Build history of the part. All positions in model axes, mm. A direction names the side the tool comes from. Round coordinates to 2 decimals unless told otherwise and drop trailing zeros. Write each loop counter-clockwise with the first axis right and the second up, starting at its lowest first coordinate (ties: lowest second). Pieces come first, ordered by that corner, then holes. Notation, with made-up numbers: (69, -11) - (75, -11) arc R26 ccw to (75, 5) - close; hole circle Ø11 at (-20, 34). An arc over 180 degrees is marked (long way). One line per question, with ' | ' between items.
from build123d import *

# Parameters (mm, degrees)
SKETCH1_W           = 1219.2
SKETCH1_H           = 508
BOSS_EXTRUDE1_DEPTH = 25.4
SKETCH2_W           = 50.8
SKETCH2_H           = 508
BOSS_EXTRUDE2_DEPTH = 304.8
SKETCH3_W           = 101.6
SKETCH3_H           = 50.8
BOSS_EXTRUDE3_DEPTH = 152.4


with BuildPart() as part:
    # Sketch1 → Boss-Extrude1 (new body)
    with BuildSketch(Plane(origin=(0, 0, 0), x_dir=(1, 0, 0), z_dir=(0, 1, 0))):
        with Locations((609.6, 254)):
            Rectangle(SKETCH1_W, SKETCH1_H)
    extrude(amount=BOSS_EXTRUDE1_DEPTH)

    # Sketch2 → Boss-Extrude2 (add)
    with BuildSketch(Plane(origin=(0, 25.4, 0), x_dir=(1, 0, 0), z_dir=(0, 1, 0))):
        with Locations((1193.8, 254)):
            Rectangle(SKETCH2_W, SKETCH2_H)
    extrude(amount=BOSS_EXTRUDE2_DEPTH)

    # Sketch3 → Boss-Extrude3 (add)
    with BuildSketch(Plane.XZ):
        with Locations((50.8, -25.4)):
            Rectangle(SKETCH3_W, SKETCH3_H)
        with Locations((50.8, -482.6)):
            Rectangle(SKETCH3_W, SKETCH3_H)
        with Locations((1168.4, -25.4)):
            Rectangle(SKETCH3_W, SKETCH3_H)
        with Locations((1168.4, -482.6)):
            Rectangle(SKETCH3_W, SKETCH3_H)
    extrude(amount=BOSS_EXTRUDE3_DEPTH)


solid = part.part
Q1. Saw through at A-A, the plane y = -114.5. List the corners of the cut face in (x, z), then the cut area to 3 significant figures.
Found:
outline: (0, -508) - (101.6, -508) - (101.6, -457.2) - (0, -457.2) - close; (0, -50.8) - (101.6, -50.8) - (101.6, 0) - (0, 0) - close; (1117.6, -508) - (1219.2, -508) - (1219.2, -457.2) - (1117.6, -457.2) - close; (1117.6, -50.8) - (1219.2, -50.8) - (1219.2, 0) - (1117.6, 0) - close | area: 20,600 mm^2
Q2. Saw through at C-C, the plane x = 364. List the corners of the cut face in (y, z), then the cut area to 3 significant figures.
Found:
outline: (0, -508) - (25.4, -508) - (25.4, 0) - (0, 0) - close | area: 12,900 mm^2
Q3. Which spindle directions (+Z, -Z, +X, -X, +Y, -Y) get a long thin tool onto all of the face, cutting with end or side? Do faces 4 (the flat face through (50, -75, -50.8)), 5 (the flat face through (1168.4, 176, -250)), 6 (the flat face through (101.6, -75, -483)). Say none if no direction does.
Found:
face 4: +X, -X, -Y | face 5: +Z, -Z, -X, +Y | face 6: +Z, -Z, -Y
Q4. Saw through at D-D, the plane y = 279. List the corners of the cut face in (x, z), then the cut area to 3 significant figures.
Found:
outline: (1168.4, -508) - (1219.2, -508) - (1219.2, 0) - (1168.4, 0) - close | area: 25,800 mm^2
Q5. Saw through at B-B, the plane z = -32. List the corners of the cut face in (x, y), then the cut area to 3 significant figures.
Found:
outline: (0, -152.4) - (101.6, -152.4) - (101.6, 0) - (1117.6, 0) - (1117.6, -152.4) - (1219.2, -152.4) - (1219.2, 330.2) - (1168.4, 330.2) - (1168.4, 25.4) - (0, 25.4) - close | area: 77,400 mm^2
Q6. Drop flat-ended pins along their axis: pin 1 (12 mm diameter, centred on x = 592, z = -457, fed in from +Y); pin 2 (5 mm diameter, centred on x = 290.5, y = 30, fed in from -Z); pin 3 (1 mm diameter, centred on y = 189, z = -349, fed in from -X); pin 4 (12 mm diameter, centred on x = 133.5, z = -154, fed in from -Y). Give the stop position or say it passes through.
Found:
pin 1: y = 25.4 | pin 2: through | pin 3: x = 1168.4 | pin 4: y = 0
Q7. Pull direction Z, two halves, no side cores. Call faces 1 (the flat face through (1168, -75, -457.2)), 2 (the flat face through (697, 1, 0)), 3 (the flat face through (101.6, -75, -26)): +Z half, -Z half, draft (parallel to the pull), parting line (faces both ways), or undercut.
Found:
face 1: undercut | face 2: +Z half | face 3: draft
Q8. Drill centre lines: L1, parallel to Y at x = 1067, z = -189; L2, parallel to X at y = 217.5, z = -110.5. Where is each one in solid material? Low to high. Write a range as from..to.
Found:
L1: 0..25.4 | L2: 1168.4..1219.2
